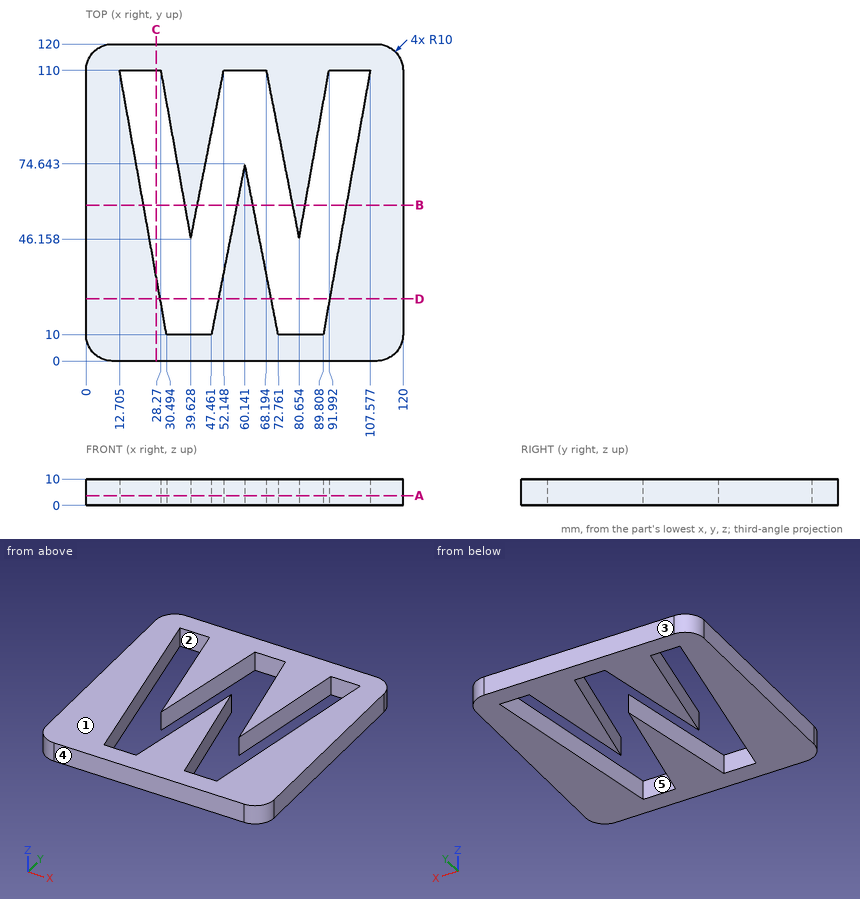
Could you check a few things on this drawing? It's one solid part, dimensions in mm from its lowest x, y, z. A direction names the side the tool comes from. Coordinates: 2 decimals unless noted, no trailing zeros. Loops run counter-clockwise (first coordinate to the right, second up) from the corner with the lowest first, then second, coordinate; pieces in that order, holes last. Notation, with made-up numbers: (5, 17) - (27, 17) arc R18 cw to (27, 37) - close; hole circle Ø8 at (31, 56). An arc over 180 degrees is marked (long way). Return JSON: item names as keys, results as strings. Group by question number.
Item 1: On a 3-axis mill with a long thin cutter (end or side, diameter ignored), from which of +Z, -Z, +X, -X, +Y, -Y can I reach the whole of each face in a straight line? I mean the marked faces 4 and 5. Say none if no direction works.
Item 2: If we section it at C-C on x = 26.5: Write out the boundary of the cut face in (y, z).
Item 3: If we section it at D-D on y = 23.5: Write out the boundary of the cut face in (x, z) (1 decimal).
Item 4: If we section it at B-B on y = 59: Write out the boundary of the cut face in (x, z) (1 decimal), and give its area (3 significant figures).
Item 5: We'd pull the mould along Y, two halves only. Please class the marked faces 1, 2 and 3: +Y half, -Y half, draft (parallel to the pull), parting line (faces both ways), or undercut.
Item 6: If we section it at A-A on z = 3.75: Write out the boundary of the cut face in (x, y) (1 decimal).
Item 7: I need wall thicknesses on line 1 (X direction, y = 19, z = 7.5) (1 decimal); line 2 (X direction, y = 104, z = 6) (1 decimal); line 3 (X direction, y = 42, z = 2.25) (1 decimal). Which ranges of each line are inside material? Lowest first, please. Write a range as from..to.
Calculated:
{
 "1": {"face 4": "+Z, -Z, +X, -X, -Y", "face 5": "+Z, -Z"},
 "2": {"outline": "(0, 0) - (32.45, 0) - (32.45, 10) - (0, 10) - close; (110, 0) - (120, 0) - (120, 10) - (110, 10) - close"},
 "3": {"outline": "(0, 0) - (28.1, 0) - (28.1, 10) - (0, 10) - close; (50.1, 0) - (70.1, 0) - (70.1, 10) - (50.1, 10) - close; (92.2, 0) - (120, 0) - (120, 10) - (92.2, 10) - close"},
 "4": {"outline": "(0, 0) - (21.8, 0) - (21.8, 10) - (0, 10) - close; (37.3, 0) - (42.1, 0) - (42.1, 10) - (37.3, 10) - close; (57.1, 0) - (63.2, 0) - (63.2, 10) - (57.1, 10) - close; (78.1, 0) - (82.9, 0) - (82.9, 10) - (78.1, 10) - close; (98.5, 0) - (120, 0) - (120, 10) - (98.5, 10) - close", "area": "590 mm^2"},
 "5": {"face 1": "draft", "face 2": "undercut", "face 3": "+Y half"},
 "6": {"outline": "(0, 10) arc R10 ccw to (10, 0) - (110, 0) arc R10 ccw to (120, 10) - (120, 110) arc R10 ccw to (110, 120) - (10, 120) arc R10 ccw to (0, 110) - close; hole (12.7, 110) - (30.5, 10) - (47.5, 10) - (60.1, 74.6) - (72.8, 10) - (89.8, 10) - (107.6, 110) - (92, 110) - (80.7, 46.2) - (68.2, 110) - (52.1, 110) - (39.6, 46.2) - (28.3, 110) - close"},
 "7": {"line 1": "x = 0..28.9, 49.2..71, 91.4..120", "line 2": "x = 0..13.8, 29.3..51, 69.4..90.9, 106.5..120", "line 3": "x = 0..24.8, 53.7..66.5, 95.5..120"}
}
